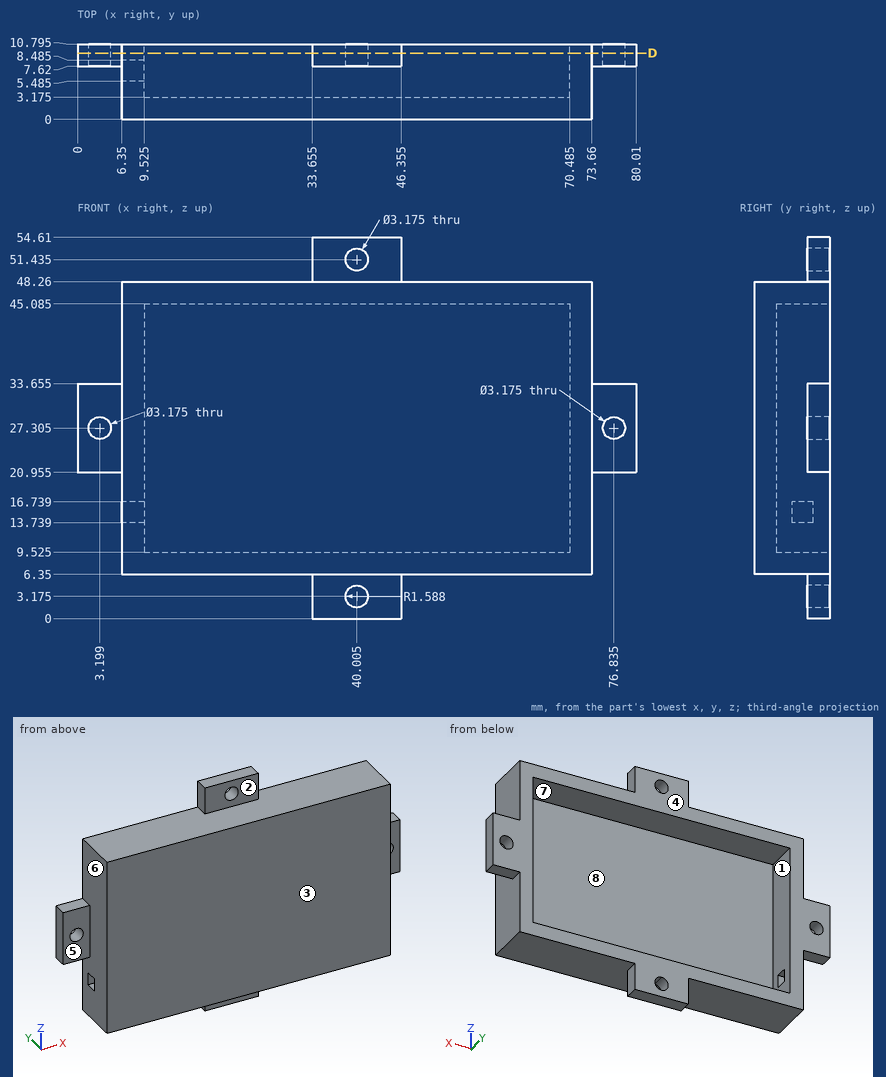
Study the drawing (mm; zero at the part's minimum x, y, z) and answer. A direction names the side the tool comes from. Give positions to 0.01 mm unless a question says otherwise; leave off trailing zeros. Return JSON: item names as keys, results as strings. Group by question number.
1. Straight lines are drawn through the part: line 1 (X direction, y = 9.5, z = 25.5) (1 decimal); line 2 (Z direction, x = 57.5, y = 1.5); line 3 (X direction, y = 5.75, z = 7). For each, find the intervals that lie inside material, in ascending order. Write a range as [from, to].
2. Given pin 1 Ø2.5 at (x, y) = (77.5, 9.5) entering from -Z (1 decimal); pin 2 Ø2 at (y, z) = (2, 41.5) entering from -X; pin 3 Ø5 at (y, z) = (9.5, 7.5) entering from +X; pin 4 Ø1.9 at (x, z) = (40.005, 51.435) entering from -Y, each flat-ended and moving along its own axis, determine where each tip first touches the part or whether it passes through.
3. Determine the mould class of the marked faces 6, 7 and 8 for opening direction Z: pulls with the +Z half, pulls with the -Z half, needs draft (parallel to the pull), parting line crosses it, or undercut.
4. Which of the six approach directions +Z, -Z, +X, -X, +Y, -Y give full straight-line access (tool end or side, diameter ignored) to the marked faces 1, 2, 3, 4 and 5?
5. Find section D-D (y = 9.5). State how many separate pieces and enclosed holes the cut face has.
Verdict:
{
 "1": {"line 1": "x = [0, 9.5], [70.5, 80]", "line 2": "z = [6.35, 48.26]", "line 3": "x = [6.35, 73.66]"},
 "2": {"pin 1": "stops at z = 21", "pin 2": "stops at x = 6.35", "pin 3": "stops at x = 73.66", "pin 4": "passes through"},
 "3": {"face 6": "needs draft", "face 7": "undercut", "face 8": "undercut"},
 "4": {"face 1": "+Y", "face 2": "+Z, +X, -X, -Y", "face 3": "+Z, -Z, +X, -X, -Y", "face 4": "+Z, -Z, +X, -X, +Y", "face 5": "+Z, -Z, -X, -Y"},
 "5": {"separate pieces": "1", "enclosed holes": "5"}
}
